Can you work these out from the model? Positions are in its coordinate system, mm. A direction names the side the tool comes from. Coordinates: 2 decimals unless noted, no trailing zeros. Loops run counter-clockwise (first coordinate to the right, second up) from the corner with the lowest first, then second, coordinate; pieces in that order, holes last. Notation, with made-up numbers: (50.5, -6.75) -> (69.5, -6.75) arc R19 cw to (69.5, 3.25) -> close; hole circle Ø3 at (43.5, 6). An arc over 180 degrees is marked (long way). Put each result on its own line as item: value. Start each with the question number.
Item 1: If we section it at C-C on x = 1: Please give me the cut outline in (y, z), plus the area to 3 significant figures.
Item 2: Will these pins go through, and if not, where does the flat tip stop? P1, Ø1.5, axis at y = -9.5, z = 5, coming from the +X side; P2, Ø4, axis at y = 5.5, z = 4, coming from the +X side; P3, Ø4.5, axis at x = 1.5, y = -1, coming from the -Z side.
Item 3: We'd pull the mould along Y, two halves only. Please class faces 1 (the cylindrical face through (-7.39, -0.13, 7.49)), 2 (the cylindrical face through (-11, 0, 8)), 3 (the cylindrical face through (-6.269, -4.807, -4.437)), 4 (the cylindrical face through (-0.07, 7.55, 6.55)): pulls with the +Y half, pulls with the -Y half, needs draft (parallel to the pull), parting line crosses it, or undercut.
Item 4: Please list where these lines run through material, in increasing order: L1, parallel to Z at x = -11, y = 6.5; L2, parallel to Z at x = 5.5, y = 0; L3, parallel to Y at x = -9.5, z = -2. Write a range as from..to.
Item 5: For faces 5 (the cylindrical face through (0.07, -7.55, 6.55)), 6 (the flat face through (-1, -9, 3)), 7 (the flat face through (-4, 2, 0)), which set-ups out of +Z, -Z, +X, -X, +Y, -Y let a thin tool reach every point of the face, with its end or its side?
Item 6: If we section it at D-D on z = 8.25: Please give me the cut outline in (x, y).
Item 7: If we section it at A-A on y = 0: Please give me the cut outline in (x, z) (3 decimals), plus the area to 3 significant figures.
Item 8: If we section it at B-B on z = -1.5: Please give me the cut outline in (x, y) (3 decimals), plus the area to 3 significant figures.
```python
from build123d import *

# Parameters (mm, degrees)
F0_R      = 14.125
F0_R_2    = 11
F0_R_3    = 4
F1_DEPTH  = 3
F2_DEPTH  = 10
F3_R      = 14.125
F3_R_2    = 7.9
F4_DEPTH  = 9
F6_DEPTH  = 12
F7_R      = 1
F8_DEPTH  = 12.5
F10_DEPTH = 7


with BuildPart() as f1:
    # F0 (on Top) → F1 (new body)
    with BuildSketch(Plane.XY):
        Circle(F0_R)
        Circle(F0_R_2, mode=Mode.SUBTRACT)
        Circle(F0_R_2)
        Circle(F0_R_3, mode=Mode.SUBTRACT)
    extrude(amount=F1_DEPTH)

    # F0 (on Top) → F2 (join)
    with BuildSketch(Plane.XY):
        Circle(F0_R_2)
        Circle(F0_R_3, mode=Mode.SUBTRACT)
    extrude(amount=F2_DEPTH)

    # F3 (on Top) → F4 (join)
    with BuildSketch(Plane.XY):
        Circle(F3_R)
        Circle(F3_R_2, mode=Mode.SUBTRACT)
    extrude(amount=-F4_DEPTH)

    # F5 (on face) → F6 (cut, through all)
    with BuildSketch(Plane.XY.offset(3)):
        with BuildLine():
            ThreePointArc((1.9373280842, 10.8280542986), (0, 11), (-1.9373280842, 10.8280542986))
            ThreePointArc((-1.9373280842, 10.8280542986), (0, 9.1), (1.9373280842, 10.8280542986))
        make_face()
        with BuildLine():
            ThreePointArc((1.9373280842, 10.8280542986), (1.9468294435, 10.9388464218), (1.95, 11.05))
            ThreePointArc((1.95, 11.05), (-0.1111535782, 12.9968294435), (-1.9373280842, 10.8280542986))
            ThreePointArc((-1.9373280842, 10.8280542986), (0, 11), (1.9373280842, 10.8280542986))
        make_face()
        with BuildLine():
            ThreePointArc((1.9373280842, -10.8280542986), (0, -9.1), (-1.9373280842, -10.8280542986))
            ThreePointArc((-1.9373280842, -10.8280542986), (0, -11), (1.9373280842, -10.8280542986))
        make_face()
        with BuildLine():
            ThreePointArc((1.9373280842, -10.8280542986), (0, -11), (-1.9373280842, -10.8280542986))
            ThreePointArc((-1.9373280842, -10.8280542986), (-0.1111535782, -12.9968294435), (1.95, -11.05))
            ThreePointArc((1.95, -11.05), (1.9468294435, -10.9388464218), (1.9373280842, -10.8280542986))
        make_face()
    extrude(amount=-F6_DEPTH, mode=Mode.SUBTRACT)

    # F7 (on Right) → F8 (cut, symmetric)
    with BuildSketch(Plane.YZ):
        with Locations((0, 6.5)):
            Circle(F7_R)
    extrude(amount=F8_DEPTH, both=True, mode=Mode.SUBTRACT)

    # F9 (on face) → F10 (cut, through all)
    with BuildSketch(Plane.XY.offset(10)):
        with BuildLine():
            ThreePointArc((3.4474570131, 10.4458144796), (0, 11), (-3.4474570131, 10.4458144796))
            ThreePointArc((-3.4474570131, 10.4458144796), (0, 7.55), (3.4474570131, 10.4458144796))
        make_face()
        with BuildLine():
            ThreePointArc((3.4474570131, -10.4458144796), (0, -7.55), (-3.4474570131, -10.4458144796))
            ThreePointArc((-3.4474570131, -10.4458144796), (0, -11), (3.4474570131, -10.4458144796))
        make_face()
    extrude(amount=-F10_DEPTH, mode=Mode.SUBTRACT)


solid = f1.part
```
Solutions:
1. outline: (-14.09, -9) -> (-12.72, -9) -> (-12.72, 3) -> (-14.09, 3) -> close; (-9.38, -9) -> (-7.84, -9) -> (-7.84, 0) -> (-3.87, 0) -> (-3.87, 10) -> (-7.7, 10) -> (-7.7, 3) -> (-9.38, 3) -> close; (3.87, 0) -> (7.84, 0) -> (7.84, -9) -> (9.38, -9) -> (9.38, 3) -> (7.7, 3) -> (7.7, 10) -> (3.87, 10) -> close; (12.72, -9) -> (14.09, -9) -> (14.09, 3) -> (12.72, 3) -> close
1. area: 147 mm^2
2. P1: x = 6.67
2. P2: x = 13.61
2. P3: z = 0
3. face 1: undercut
3. face 2: parting line crosses it
3. face 3: undercut
3. face 4: pulls with the +Y half
4. L1: -9..3
4. L2: 0..5.5, 7.5..10
4. L3: -10.45..10.45
5. face 5: +Z, -Y
5. face 6: +Z
5. face 7: -Z
6. outline: (-3.45, -10.45) arc R3.5 cw to (3.45, -10.45) arc R11 ccw to (3.45, 10.45) arc R3.5 cw to (-3.45, 10.45) arc R11 ccw to start; hole circle Ø8 at (0, 0)
7. outline: (-14.125, -9) -> (-7.9, -9) -> (-7.9, 0) -> (-4, 0) -> (-4, 5.5) -> (-11, 5.5) -> (-11, 3) -> (-14.125, 3) -> close; (-11, 7.5) -> (-4, 7.5) -> (-4, 10) -> (-11, 10) -> close; (4, 0) -> (7.9, 0) -> (7.9, -9) -> (14.125, -9) -> (14.125, 3) -> (11, 3) -> (11, 5.5) -> (4, 5.5) -> close; (4, 7.5) -> (11, 7.5) -> (11, 10) -> (4, 10) -> close
7. area: 243 mm^2
8. outline: circle Ø28.25 at (0, 0); hole circle Ø15.8 at (0, 0); hole circle Ø3.9 at (0, -11.05); hole circle Ø3.9 at (0, 11.05)
8. area: 407 mm^2
